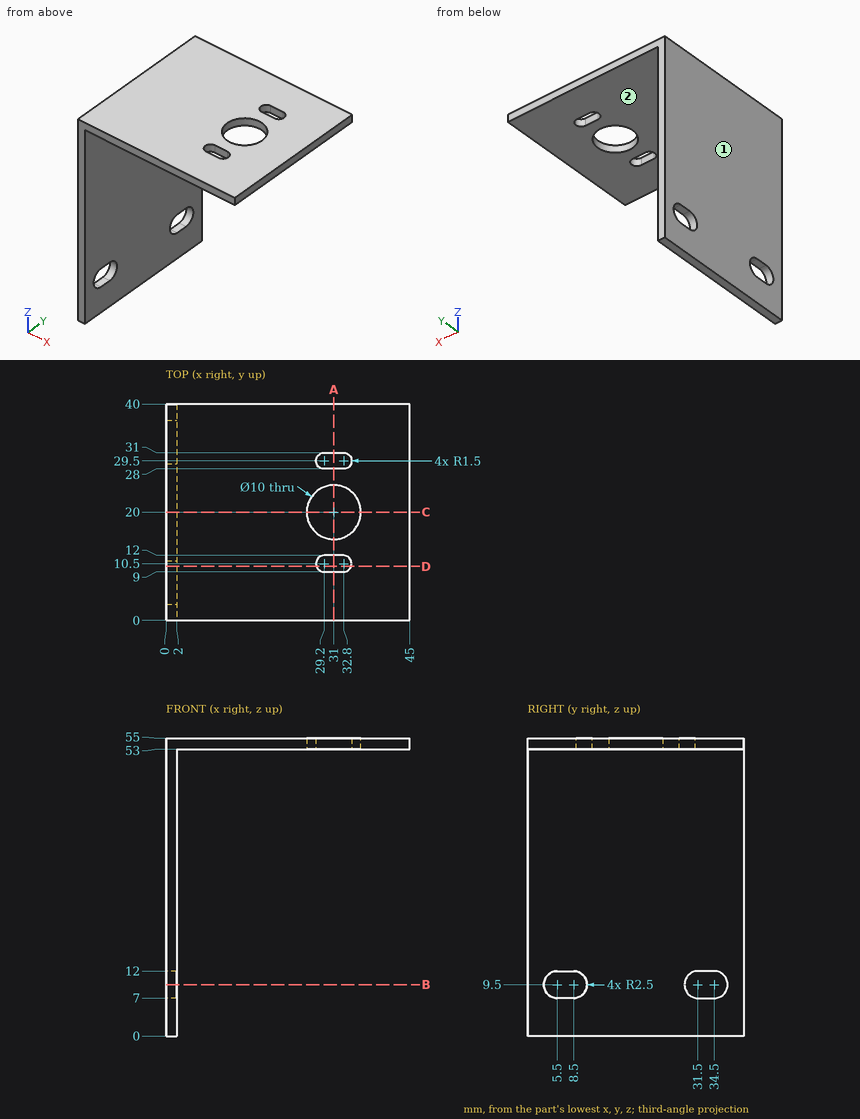
Design review of the part shown in the three views and the two pictorial views. Dimensions are in mm from the part's minimum x, y and z. A direction names the side the tool comes from. Coordinates: 2 decimals unless noted, no trailing zeros. Order: outer loops, then holes, each group sorted by start corner. A loop starts at its lowest first (then second) coordinate and runs counter-clockwise, first axis right, second up.
Item 1: For the marked faces 1 and 2, list the 3-axis set-ups (+Z, -Z, +X, -X, +Y, -Y) from which the entire face can be reached by the end or side of a thin tool; tool diameter is ignored.
Item 2: Take a section at A-A, the plane x = 31. Write out the cut boundary in (y, z).
Item 3: For line 1 (Y direction, x = 31, z = 53.95); line 2 (Z direction, x = 9, y = 30); line 3 (X direction, y = 8, z = 47), list the stretches that pass through material, from the lowest coordinate up.
Item 4: Take a section at D-D, the plane y = 10. Write out the cut boundary in (x, z).
Item 5: For pin 1 Ø5 at (x, z) = (18, 48.5) entering from +Y; pin 2 Ø12 at (y, z) = (33.5, 16.5) entering from +X; pin 3 Ø10 at (x, y) = (22.5, 4.5) entering from -Z, all flat-tipped, find the tip position at first contact; note any pin that passes through.
Item 6: Take a section at C-C, the plane y = 20. Write out the cut boundary in (x, z), then the cut area to 3 significant figures.
Item 7: Take a section at B-B, the plane z = 9.5. Write out the cut boundary in (x, y).
The answers:
1. face 1: +Z, -Z, -X, +Y, -Y
1. face 2: -Z, +X, +Y, -Y
2. outline: (0, 53) - (9, 53) - (9, 55) - (0, 55) - close; (12, 53) - (15, 53) - (15, 55) - (12, 55) - close; (25, 53) - (28, 53) - (28, 55) - (25, 55) - close; (31, 53) - (40, 53) - (40, 55) - (31, 55) - close
3. line 1: y = 0 to 9, 12 to 15, 25 to 28, 31 to 40
3. line 2: z = 53 to 55
3. line 3: x = 0 to 2
4. outline: (0, 0) - (2, 0) - (2, 7.5) - (0, 7.5) - close; (0, 11.5) - (2, 11.5) - (2, 53) - (27.79, 53) - (27.79, 55) - (0, 55) - close; (34.21, 53) - (45, 53) - (45, 55) - (34.21, 55) - close
5. pin 1: passes through
5. pin 2: stops at x = 2
5. pin 3: stops at z = 53
6. outline: (0, 0) - (2, 0) - (2, 53) - (26, 53) - (26, 55) - (0, 55) - close; (36, 53) - (45, 53) - (45, 55) - (36, 55) - close
6. area: 176 mm2
7. outline: (0, 0) - (2, 0) - (2, 3) - (0, 3) - close; (0, 11) - (2, 11) - (2, 29) - (0, 29) - close; (0, 37) - (2, 37) - (2, 40) - (0, 40) - close
